Autodesk Inventor part; units mm, degrees
ref_plane "YZ Plane" through (0, 0, 0) normal (1, 0, 0) x (0, 1, 0)
ref_plane "XZ Plane" through (0, 0, 0) normal (0, 1, 0) x (-1, 0, 0)
ref_plane "XY Plane" through (0, 0, 0) normal (0, 0, 1) x (1, 0, 0)
sketch "スケッチ1" plane through (0, 0, 0) normal (0, 0, 1) x (1, 0, 0)
  line L0 (0, 3.1754) -> (2.75, 1.5877)
  line L1 (2.75, 1.5877) -> (2.75, -1.5877)
  line L2 (2.75, -1.5877) -> (0, -3.1754)
  line L3 (0, -3.1754) -> (-2.75, -1.5877)
  line L4 (-2.75, -1.5877) -> (-2.75, 1.5877)
  line L5 (-2.75, 1.5877) -> (0, 3.1754)
  point P0 (0, 0)
  point P1 (0, 0)
  dimension "d0" = 5.5
extrude "押し出し1" add sketch "スケッチ1" along normal blind 5
sketch "スケッチ2" plane through (0, 0, 5) normal (0, 0, 1) x (1, 0, 0)
  circle A0 centre (0, 0) radius 1.5
  dimension "d3" = 3
extrude "押し出し2" add sketch "スケッチ2" along normal blind 5
thread "ねじ1"
chamfer "面取り1" distance 0.3 angle 45 1 edges at (-1.5, 0, 10)
fillet "フィレット1" radius 0.2 18 edges at (-1.375, 2.3816, 5) (1.375, 2.3816, 5) (2.75, 0, 5) (1.375, -2.3816, 5) (-1.375, -2.3816, 5) (-2.75, 0, 5) (-2.75, -1.5877, 2.5) (0, -3.1754, 2.5) (2.75, -1.5877, 2.5) (2.75, 1.5877, 2.5) (0, 3.1754, 2.5) (-2.75, 1.5877, 2.5) (-1.375, 2.3816, 0) (1.375, 2.3816, 0) (2.75, 0, 0) (1.375, -2.3816, 0) (-1.375, -2.3816, 0) (-2.75, 0, 0)
sketch "スケッチ3" plane through (0, 0, 0) normal (0, 0, -1) x (-1, 0, 0)
  point P0 (0, 0)
hole "穴1" at (0, 0, 0) direction (0, 0, 1) diameter 2.459 depth 5 tip angle 118
chamfer "面取り2" distance 0.2 angle 45 1 edges at (0, -1.2295, 0)
properties part number "hexagonal_spacer_M3_5mm" material "鋼、炭素鋼"
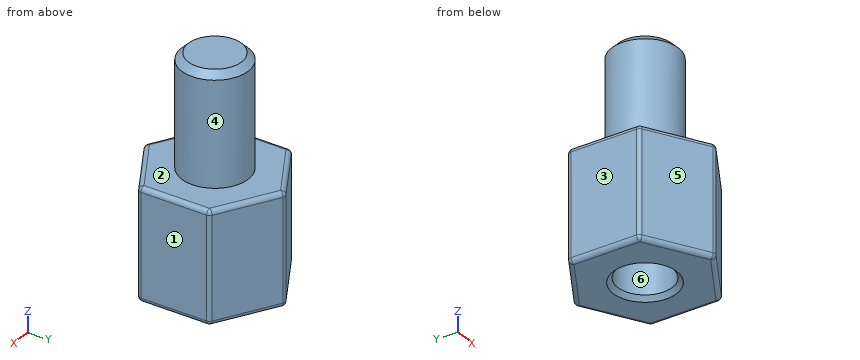
Model file for the job. Use its own axes, mm. Face numbers are marked on the shaded views. A direction names the side the tool comes from. Give positions to 0.01 mm unless a question says otherwise; leave off trailing zeros. Loops run counter-clockwise (first coordinate to the right, second up) from the corner with the lowest first, then second, coordinate; pieces in that order, holes last.
1) Flat gauge pins, fed straight in: pin 1 Ø2 at (y, z) = (1.5, 7) entering from -X; pin 2 Ø1.5 at (x, y) = (0.5, -1.5) entering from +Z. Where does each tip first touch, or does it go through?
2) Pull direction Y, two halves, no side cores. Call the marked faces 3, 4, 5 and 6: +Y half, -Y half, draft (parallel to the pull), parting line (faces both ways), or undercut.
3) Saw through at B-B (z = 7.75). Write the cut outline in (x, y), plus the area to 3 significant figures.
4) Tool access for the marked faces 1 and 2: list every direction of +Z, -Z, +X, -X, +Y, -Y with a clear straight run to the whole face (end or side of a thin tool).
5) Saw through at A-A (z = 2). Write the cut outline in (x, y), plus the area to 3 significant figures.
6) Wall check: line 1 (Y direction, x = 0, z = 3.5); line 2 (X direction, y = 0, z = 2.45); line 3 (Z direction, x = -0.2, y = -2.5). Give the ranges that are in metal, low to high.
Answer block:
1. pin 1: stops at x = -1.41
1. pin 2: stops at z = 10
2. face 3: draft
2. face 4: parting line
2. face 5: -Y half
2. face 6: undercut
3. outline: circle Ø3 at (0, 0)
3. area: 7.07 mm2
4. face 1: +Z, -Z, +X, +Y, -Y
4. face 2: +Z
5. outline: (-2.75, -1.47) arc R0.2 ccw to (-2.65, -1.65) - (-0.1, -3.12) arc R0.2 ccw to (0.1, -3.12) - (2.65, -1.65) arc R0.2 ccw to (2.75, -1.47) - (2.75, 1.47) arc R0.2 ccw to (2.65, 1.65) - (0.1, 3.12) arc R0.2 ccw to (-0.1, 3.12) - (-2.65, 1.65) arc R0.2 ccw to (-2.75, 1.47) - close; hole circle Ø2.46 at (0, 0)
5. area: 21.4 mm2
6. line 1: y = -3.14 to -1.23, 1.23 to 3.14
6. line 2: x = -2.75 to -1.23, 1.23 to 2.75
6. line 3: z = 0 to 5
